Can you work these out from the model? Positions are in its coordinate system, mm. A direction names the side the tool comes from. Round coordinates to 2 decimals unless told otherwise and drop trailing zeros. Write each loop counter-clockwise with the first axis right and the second up, starting at its lowest first coordinate (ties: lowest second). Pieces come first, ordered by that corner, then holes.
Q1. Please list where these lines run through material, in increasing order: line 1 along X through (y, z) = (12, 1.75); line 2 along X through (y, z) = (9, 0.6); line 3 along X through (y, z) = (-9, 1.1).
Q2. I'm going to push flat-ended pins straight in: pin 1 Ø1.5 at (x, z) = (0, 0.5) entering from -Y; pin 2 Ø4 at (x, y) = (24.91, 24.76) entering from +Z; pin 3 Ø0.9 at (y, z) = (12.5, 2) entering from -X; pin 4 Ø1 at (y, z) = (-10, 1) entering from -X. Where does each tip first touch, or does it pass through?
Q3. If we section it at A-A (x = -12): Please give me the cut outline in (y, z), plus the area to 3 significant figures.
Q4. If we section it at D-D (y = 3): Please give me the cut outline in (x, z).
Q5. We'd pull the mould along Y, two halves only. Please class faces 1 (the cylindrical face through (7.73, 6.48, 1.52)), 2 (the cylindrical face through (-8.585, 9.255, 1.521)), 3 (the flat face through (21.463, 25, 1)), 4 (the cylindrical face through (20.89, 22.61, 1.52)): +Y half, -Y half, draft (parallel to the pull), parting line (faces both ways), or undercut.
Q6. For faces 5 (the flat face through (-12, 16.013, 1)), 6 (the flat face through (12.232, 10.536, 1.479)), 7 (the flat face through (2.658, -5.625, 1.479)), which set-ups out of +Z, -Z, +X, -X, +Y, -Y let a thin tool reach every point of the face, with its end or its side?
Q7. If we section it at B-B (x = 3): Please give me the cut outline in (y, z), plus the area to 4 significant figures.
Q8. If we section it at C-C (z = 1.6): Give the number of separate pieces and of enclosed holes in the cut face, plus the area to 3 significant figures.
from build123d import *

# Parameters (mm, degrees)
F0_R        = 3.95
F0_R_2      = 1.25
F0_R_3      = 1.5
F1_DEPTH    = 3
F2_R        = 10
F3_R        = 2
F4_T1_DEPTH = 16.2671931878
F4_T3_DEPTH = 33.1863063341


# Not quite as in the source:
# - a fillet or chamfer that OpenCascade refuses, or shapes differently, is made with other operations: its cross-section is extruded or revolved along the edge and cut away or added
# - a feature names something its author has since deleted; it is built from what else it names


with BuildPart() as f1:
    # F0 (on Top) → F1 (new body)
    with BuildSketch(Plane.XY):
        with BuildLine():
            Line((4.0200765709, -14.8563961814), (9.9142113018, -14.8563961814))
            Line((9.9142113018, -14.8563961814), (9.9142113018, -11.4412054596))
            Line((9.9142113018, -11.4412054596), (9.9142113018, 0))
            Line((9.9142113018, 0), (21.4632351379, 17.0130324811))
            Line((21.4632351379, 17.0130324811), (28.3592351379, 17.0130324811))
            Line((28.3592351379, 17.0130324811), (28.3592351379, 22.0130324811))
            Line((28.3592351379, 22.0130324811), (28.3592351379, 27.5130324811))
            Line((28.3592351379, 27.5130324811), (21.4632351379, 27.5130324811))
            Line((21.4632351379, 27.5130324811), (21.4632351379, 22.0130324811))
            Line((21.4632351379, 22.0130324811), (-8.7310690433, 22.0130324811))
            Line((-8.7310690433, 22.0130324811), (-14.7310690433, 22.0130324811))
            Line((-14.7310690433, 22.0130324811), (-14.7310690433, 16.0130324811))
            Line((-14.7310690433, 16.0130324811), (-8.7310690433, 16.0130324811))
            Line((-8.7310690433, 16.0130324811), (-8.7310690433, 9.2081045732))
            Line((-8.7310690433, 9.2081045732), (0, 0))
            Line((0, 0), (0, -4.9987894588))
            Line((0, -4.9987894588), (3.805913418, -5.8956493604))
            ThreePointArc((3.805913418, -5.8956493604), (6.3099596188, -9.1166975853), (3.693151613, -12.2468277588))
            ThreePointArc((3.693151613, -12.2468277588), (3.0604717322, -12.3090046508), (2.4277918514, -12.2468277588))
            Line((2.4277918514, -12.2468277588), (0, -12.2468277588))
            Line((0, -12.2468277588), (0, -13.2468277588))
            Line((0, -13.2468277588), (4.0200765709, -14.8563961814))
        make_face()
        with Locations((0, 12.3804118484)):
            Circle(F0_R, mode=Mode.SUBTRACT)
        with Locations((-11.7310690433, 19.0130324811)):
            Circle(F0_R_2, mode=Mode.SUBTRACT)
        Polygon((6.3511028036, 16.8475485612), (16.5163309854, 16.8475485612), (6.3511028036, 1.8730052848), align=None, mode=Mode.SUBTRACT)
        with Locations((24.9112351379, 24.7630324811)):
            Circle(F0_R_3, mode=Mode.SUBTRACT)
    extrude(amount=F1_DEPTH)

    # F2
    f2_edges = [f1.edges().sort_by_distance(p)[0] for p in [
        (4.020077, -14.856396, 1.5),
    ]]
    fillet(f2_edges, radius=F2_R)

    # F3
    f3_edges = [f1.edges().sort_by_distance(p)[0] for p in [
        (21.463235, 22.013032, 1.5),
        (-8.731069, 9.208105, 1.5),
        (21.463235, 17.013032, 1.5),
        (0, 0, 1.5),
        (0, -4.998789, 1.5),
        (9.914211, 0, 1.5),
        (6.351103, 16.847549, 1.5),
        (16.516331, 16.847549, 1.5),
        (6.351103, 1.873005, 1.5),
        (-14.731069, 16.013032, 1.5),
        (-14.731069, 22.013032, 1.5),
        (28.359235, 27.513032, 1.5),
        (21.463235, 27.513032, 1.5),
        (28.359235, 17.013032, 1.5),
        (-8.731069, 16.013032, 1.5),
    ]]
    fillet(f3_edges, radius=F3_R)

    # F4: fillet of radius 5 on 2 edges, made by hand

    # F4_s2 → F4_t1 (cut)
    with BuildSketch(Plane.XY.offset(-6.6335965939)):
        with BuildLine():
            ThreePointArc((2.4644968667, -14.2301851696), (1.0712579431, -13.4385513762), (0, -12.2468277588))
            Line((0, -12.2468277588), (-0.4206053642, -12.5171814672))
            ThreePointArc((-0.4206053642, -12.5171814672), (-0.5, -12.7468277588), (-0.5, -13.2468277588))
            Line((-0.5, -13.2468277588), (-0.1858483979, -13.7110048511))
            ThreePointArc((-0.1858483979, -13.7110048511), (2.0447940609, -14.6041151192), (2.2903411892, -14.698874619))
            Line((2.2903411892, -14.698874619), (2.4644968667, -14.2301851696))
        make_face()
    extrude(amount=F4_T1_DEPTH, mode=Mode.SUBTRACT)

    # F4_s4 → F4_t3 (cut)
    with BuildSketch(Plane.XY.offset(-15.0931531671)):
        with BuildLine():
            ThreePointArc((9.9142113018, -9.7484393403), (8.063259128, -13.6321872452), (3.8808121864, -14.6404824992))
            Line((3.8808121864, -14.6404824992), (3.7774722749, -15.1296868151))
            ThreePointArc((3.7774722749, -15.1296868151), (5.9476104172, -15.3563961814), (9.9142113018, -15.3563961814))
            Line((9.9142113018, -15.3563961814), (10.4142113018, -14.8563961814))
            Line((10.4142113018, -14.8563961814), (10.4142113018, -9.7484393403))
            Line((10.4142113018, -9.7484393403), (9.9142113018, -9.7484393403))
        make_face()
    extrude(amount=F4_T3_DEPTH, mode=Mode.SUBTRACT)


solid = f1.part
A:
1. line 1: x = -8.73 to -3.93, 3.93 to 6.35, 13.23 to 18.06
1. line 2: x = -8.46 to -2.04, 2.04 to 6.35, 11.19 to 16.02
1. line 3: x = 6.31 to 9.91
2. pin 1: stops at y = -13.16
2. pin 2: stops at z = 3
2. pin 3: stops at x = -8.73
2. pin 4: stops at x = 5.97
3. outline: (16.01, 0) - (17.79, 0) - (17.79, 3) - (16.01, 3) - close; (20.23, 0) - (22.01, 0) - (22.01, 3) - (20.23, 3) - close
3. area: 10.7 mm2
4. outline: (-2.84, 0) - (11.95, 0) - (11.95, 3) - (-2.84, 3) - close
5. face 1: undercut
5. face 2: -Y half
5. face 3: draft
5. face 4: +Y half
6. face 5: +Z, -Z, -X, -Y
6. face 6: +Z, -Z
6. face 7: +Z, -Z, -X
7. outline: (-14.41, 0) - (-12.31, 0) - (-12.31, 3) - (-14.41, 3) - close; (-5.71, 0) - (9.81, 0) - (9.81, 3) - (-5.71, 3) - close; (14.95, 0) - (22.01, 0) - (22.01, 3) - (14.95, 3) - close
7. area: 74.05 mm2
8. separate pieces: 1
8. enclosed holes: 4
8. area: 606 mm2
